```python
from build123d import *

# Parameters (mm, degrees)
BOSS_EXTRUDE1_DEPTH = 550
SKETCH2_W           = 550
SKETCH2_H           = 2.1
SKETCH3_W           = 550
SKETCH3_H           = 2.1
SKETCH4_W           = 550
SKETCH4_H           = 2.1


with BuildPart() as part:
    # Sketch1 → Boss-Extrude1 (new body)
    with BuildSketch(Plane.XY):
        with BuildLine():
            Line((-10, -17), (-8, -17))
            Line((-8, -17), (-8, -14))
            Line((-8, -14), (-7.060660172, -14))
            Line((-7.060660172, -14), (-4, -17.060660172))
            Line((-4, -17.060660172), (-4, -19.480384758))
            Line((-4, -19.480384758), (-3.7, -20))
            Line((-3.7, -20), (-4, -20.519615242))
            Line((-4, -20.519615242), (-4, -22.939339828))
            Line((-4, -22.939339828), (-7.060660172, -26))
            Line((-7.060660172, -26), (-8, -26))
            Line((-8, -26), (-8, -23))
            Line((-8, -23), (-10, -23))
            Line((-10, -23), (-10, -29))
            ThreePointArc((-10, -29), (-9.707106781, -29.707106781), (-9, -30))
            Line((-9, -30), (-3, -30))
            Line((-3, -30), (-3, -28))
            Line((-3, -28), (-6, -28))
            Line((-6, -28), (-6, -27.060660172))
            Line((-6, -27.060660172), (-2.939339828, -24))
            Line((-2.939339828, -24), (-0.519615242, -24))
            Line((-0.519615242, -24), (0, -23.7))
            Line((0, -23.7), (0.519615242, -24))
            Line((0.519615242, -24), (2.939339828, -24))
            Line((2.939339828, -24), (6, -27.060660172))
            Line((6, -27.060660172), (6, -28))
            Line((6, -28), (3, -28))
            Line((3, -28), (3, -30))
            Line((3, -30), (9, -30))
            ThreePointArc((9, -30), (9.707106781, -29.707106781), (10, -29))
            Line((10, -29), (10, -23))
            Line((10, -23), (8, -23))
            Line((8, -23), (8, -26))
            Line((8, -26), (7.060660172, -26))
            Line((7.060660172, -26), (4, -22.939339828))
            Line((4, -22.939339828), (4, -20.519615242))
            Line((4, -20.519615242), (3.7, -20))
            Line((3.7, -20), (4, -19.480384758))
            Line((4, -19.480384758), (4, -17.060660172))
            Line((4, -17.060660172), (7.060660172, -14))
            Line((7.060660172, -14), (8, -14))
            Line((8, -14), (8, -17))
            Line((8, -17), (10, -17))
            Line((10, -17), (10, -3))
            Line((10, -3), (8, -3))
            Line((8, -3), (8, -6))
            Line((8, -6), (7.060660172, -6))
            Line((7.060660172, -6), (4, -2.939339828))
            Line((4, -2.939339828), (4, -0.519615242))
            Line((4, -0.519615242), (3.7, 0))
            Line((3.7, 0), (4, 0.519615242))
            Line((4, 0.519615242), (4, 2.939339828))
            Line((4, 2.939339828), (7.060660172, 6))
            Line((7.060660172, 6), (8, 6))
            Line((8, 6), (8, 3))
            Line((8, 3), (10, 3))
            Line((10, 3), (10, 17))
            Line((10, 17), (8, 17))
            Line((8, 17), (8, 14))
            Line((8, 14), (7.060660172, 14))
            Line((7.060660172, 14), (4, 17.060660172))
            Line((4, 17.060660172), (4, 19.480384758))
            Line((4, 19.480384758), (3.7, 20))
            Line((3.7, 20), (4, 20.519615242))
            Line((4, 20.519615242), (4, 22.939339828))
            Line((4, 22.939339828), (7.060660172, 26))
            Line((7.060660172, 26), (8, 26))
            Line((8, 26), (8, 23))
            Line((8, 23), (10, 23))
            Line((10, 23), (10, 29))
            ThreePointArc((10, 29), (9.707106781, 29.707106781), (9, 30))
            Line((9, 30), (3, 30))
            Line((3, 30), (3, 28))
            Line((3, 28), (6, 28))
            Line((6, 28), (6, 27.060660172))
            Line((6, 27.060660172), (2.939339828, 24))
            Line((2.939339828, 24), (0.519615242, 24))
            Line((0.519615242, 24), (0, 23.7))
            Line((0, 23.7), (-0.519615242, 24))
            Line((-0.519615242, 24), (-2.939339828, 24))
            Line((-2.939339828, 24), (-6, 27.060660172))
            Line((-6, 27.060660172), (-6, 28))
            Line((-6, 28), (-3, 28))
            Line((-3, 28), (-3, 30))
            Line((-3, 30), (-9, 30))
            ThreePointArc((-9, 30), (-9.707106781, 29.707106781), (-10, 29))
            Line((-10, 29), (-10, 23))
            Line((-10, 23), (-8, 23))
            Line((-8, 23), (-8, 26))
            Line((-8, 26), (-7.060660172, 26))
            Line((-7.060660172, 26), (-4, 22.939339828))
            Line((-4, 22.939339828), (-4, 20.519615242))
            Line((-4, 20.519615242), (-3.7, 20))
            Line((-3.7, 20), (-4, 19.480384758))
            Line((-4, 19.480384758), (-4, 17.060660172))
            Line((-4, 17.060660172), (-7.060660172, 14))
            Line((-7.060660172, 14), (-8, 14))
            Line((-8, 14), (-8, 17))
            Line((-8, 17), (-10, 17))
            Line((-10, 17), (-10, 3))
            Line((-10, 3), (-8, 3))
            Line((-8, 3), (-8, 6))
            Line((-8, 6), (-7.060660172, 6))
            Line((-7.060660172, 6), (-4, 2.939339828))
            Line((-4, 2.939339828), (-4, 0.519615242))
            Line((-4, 0.519615242), (-3.7, 0))
            Line((-3.7, 0), (-4, -0.519615242))
            Line((-4, -0.519615242), (-4, -2.939339828))
            Line((-4, -2.939339828), (-7.060660172, -6))
            Line((-7.060660172, -6), (-8, -6))
            Line((-8, -6), (-8, -3))
            Line((-8, -3), (-10, -3))
            Line((-10, -3), (-10, -17))
        make_face()
        Polygon((-8, 8), (-6.939339828, 8), (-2.939339828, 4), (2.939339828, 4), (6.939339828, 8), (8, 8), (8, 12), (6.939339828, 12), (2.939339828, 16), (-2.939339828, 16), (-6.939339828, 12), (-8, 12), align=None, mode=Mode.SUBTRACT)
        Polygon((-8, -8), (-8, -12), (-6.939339828, -12), (-2.939339828, -16), (2.939339828, -16), (6.939339828, -12), (8, -12), (8, -8), (6.939339828, -8), (2.939339828, -4), (-2.939339828, -4), (-6.939339828, -8), align=None, mode=Mode.SUBTRACT)
    extrude(amount=-BOSS_EXTRUDE1_DEPTH)

    # Sketch2 → Cut-Revolve1 (revolve, cut)
    with BuildSketch(Plane(origin=(0, 0, 0), x_dir=(0, 0, -1), z_dir=(1, 0, 0)), mode=Mode.PRIVATE) as cut_revolve1_sk:
        with Locations((275, 18.95)):
            Rectangle(SKETCH2_W, SKETCH2_H)
    revolve(cut_revolve1_sk.sketch.rotate(Axis((0, 20, 0), (0, 0, -1)), 90), axis=Axis((0, 20, 0), (0, 0, -1)), mode=Mode.SUBTRACT)

    # Sketch3 → Cut-Revolve2 (revolve, cut)
    with BuildSketch(Plane(origin=(0, 0, 0), x_dir=(0, 0, -1), z_dir=(1, 0, 0)), mode=Mode.PRIVATE) as cut_revolve2_sk:
        with Locations((275, -1.05)):
            Rectangle(SKETCH3_W, SKETCH3_H)
    revolve(cut_revolve2_sk.sketch.rotate(Axis((0, 0, 0), (0, 0, -1)), 90), axis=Axis((0, 0, 0), (0, 0, -1)), mode=Mode.SUBTRACT)

    # Sketch4 → Cut-Revolve3 (revolve, cut)
    with BuildSketch(Plane(origin=(0, 0, 0), x_dir=(0, 0, -1), z_dir=(1, 0, 0)), mode=Mode.PRIVATE) as cut_revolve3_sk:
        with Locations((275, -21.05)):
            Rectangle(SKETCH4_W, SKETCH4_H)
    revolve(cut_revolve3_sk.sketch.rotate(Axis((0, -20, 0), (0, 0, -1)), 90), axis=Axis((0, -20, 0), (0, 0, -1)), mode=Mode.SUBTRACT)


solid = part.part
```
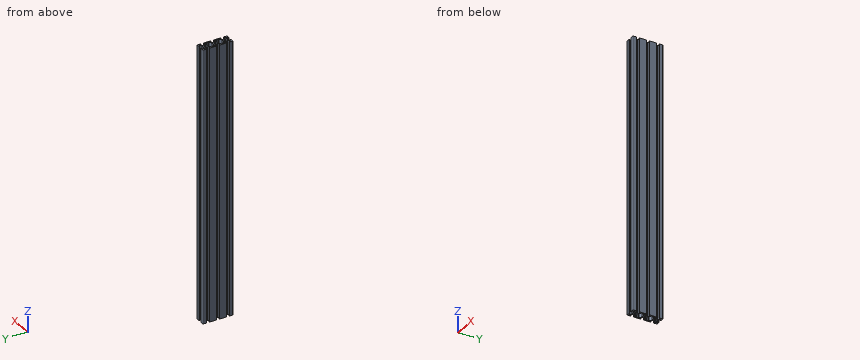
Part model, mm, in its own coordinate system. Round coordinates to 2 decimals unless told otherwise and drop trailing zeros. Answer in a Markdown table with one row per item. Add a question column.
Q1. Cut at A-A on z = -496. Give the number of separate pieces and of enclosed holes in the cut face, and give its area (3 significant figures).
Q2. Pin check, flat tips, straight feed: pin 1 (2.5 mm diameter, centred on y = 18.5, z = -241, fed in from +X); pin 2 (1.9 mm diameter, centred on y = -1.5, z = -341.5, fed in from -X); pin 3 (1 mm diameter, centred on x = 7.5, y = -1.5, fed in from +Z). Stop position of each tip, or through.
Q3. Wall check: L1, parallel to Y at x = 2.5, z = -254.5; L2, parallel to Y at x = -7, z = -496.5; L3, parallel to Y at x = 0, z = -322.5. Give the ranges that are in metal, low to high. Write a range as from..to.
Established:
| question | item | result |
|---|---|---|
| 1 | separate pieces | 1 |
| 1 | enclosed holes | 5 |
| 1 | area | 465 mm2 |
| 2 | pin 1 | stops at x = 4 |
| 2 | pin 2 | stops at x = -4 |
| 2 | pin 3 | passes through |
| 3 | L1 | y = -24..-16, -4..4, 16..24 |
| 3 | L2 | y = -30..-25.94, -14.06..-12, -8..-5.94, 5.94..8, 12..14.06, 25.94..30 |
| 3 | L3 | y = -23.7..-22.1, -17.9..-16, -4..-2.1, 2.1..4, 16..17.9, 22.1..23.7 |
